Read the model definition and answer for the solid it produces. Units are mm, in the model's axes. Face numbers are marked on the shaded views. Coordinates: 2 decimals unless noted, no trailing zeros. Loops run counter-clockwise (first coordinate to the right, second up) from the corner with the lowest first, then second, coordinate; pieces in that order, holes last. Notation, with made-up numbers: (38.5, -8.5) -> (84.5, -8.5) arc R23 ccw to (84.5, 4.5) -> close; hole circle Ø11 at (14.5, -25). An arc over 180 degrees is marked (long way). Answer as a JSON object with one key per item and string values. Group by question number.
1) Flat-ended cylindrical pins translate along their axes: P1, Ø1.5, axis at y = 5.5, z = 7.5, coming from the -X side; P2, Ø2, axis at x = 5, y = 1, coming from the +Z side. Find the tip coordinate at first contact, or state that the pin passes through.
2) Determine the mould class of the marked faces 1, 2 and 3 for opening direction X: released by +X, released by -X, zero draft, split by the parting line, or undercut.
3) Section D-D, the plane z = 7.5 is taken. Give the vertices of the cut face in (x, y), plus the area to 3 significant figures.
4) Section C-C, the plane y = 1.75 is taken. Give the vertices of the cut face in (x, z), plus the area to 3 significant figures.
5) Section B-B, the plane z = 0 is taken. Give the vertices of the cut face in (x, y).
6) Consider probe 1 along Z at (x, y) = (0, 3.25); probe 2 along X at (y, z) = (5.25, 0.5); probe 3 along Z at (x, y) = (1.25, 2). Determine where each line is inside the solid, lowest interval first. Write a range as [from, to].
7) Section A-A, the plane x = 8 is taken. Give the vertices of the cut face in (y, z).
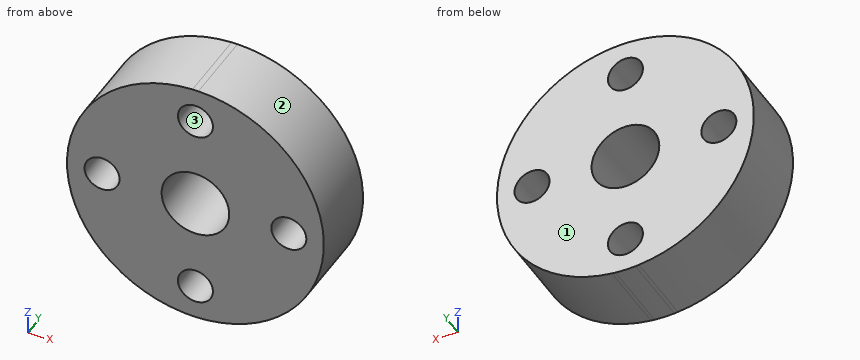
Autodesk Inventor part; units mm, degrees
ref_plane "YZ Plane" through (0, 0, 0) normal (1, 0, 0) x (0, 1, 0)
ref_plane "XZ Plane" through (0, 0, 0) normal (0, 1, 0) x (-1, 0, 0)
ref_plane "XY Plane" through (0, 0, 0) normal (0, 0, 1) x (1, 0, 0)
sketch "Эскиз1" plane through (0, 0, 0) normal (0, 1, 0) x (-1, 0, 0)
  arc A0 (-0.25, 9.2247) -> (0.25, 9.2247) centre (0, 8) ccw
  line L0 (-0.25, 10.9972) -> (-0.25, 9.2247)
  arc A1 (-0.25, 10.9972) -> (-1.1469, -10.94) centre (0, 0) ccw
  line L1 (-1.1469, -10.6297) -> (-1.1469, -10.94)
  line L2 (-0.8473, -10.6297) -> (-1.1469, -10.6297)
  line L3 (-0.8473, -10.9673) -> (-0.8473, -10.6297)
  arc A2 (-0.8473, -10.9673) -> (0.8535, -10.9668) centre (0, 0) ccw
  line L4 (0.8535, -10.6297) -> (0.8535, -10.9668)
  line L5 (1.1541, -10.6297) -> (0.8535, -10.6297)
  line L6 (1.1541, -10.9393) -> (1.1541, -10.6297)
  arc A3 (1.1541, -10.9393) -> (0.25, 10.9972) centre (0, 0) ccw
  line L7 (0.25, 9.2247) -> (0.25, 10.9972)
  circle A4 centre (8, 0) radius 1.25
  circle A5 centre (0, -8) radius 1.25
  circle A6 centre (-8, 0) radius 1.25
  circle A7 centre (0, -5.5) radius 0.75
  circle A8 centre (4.7631, 2.75) radius 0.75
  circle A9 centre (-4.7631, 2.75) radius 0.75
  circle A10 centre (0, 0) radius 2.9
  arc A11 (0.25, 9.2247) -> (-0.25, 9.2247) centre (0, 8) ccw
  line L8 (0.25, 10.9972) -> (-0.25, 10.9972)
  line L9 (1.1541, -10.9393) -> (0.8535, -10.9668)
  line L10 (-0.8473, -10.9673) -> (-1.1541, -10.9393)
extrude "Выдавливание1" add sketch "Эскиз1" along normal blind 6.5 contours A0 L7 A3 L6 L5 L4 A2 L3 L2 L1 A1 L0 | L0 L8 L7 A11 | L9 L4 L5 L6 | L1 L2 L3 L10 | A7 | A8 | A9
sketch "Эскиз2" plane through (0, 6.5, 0) normal (0, 1, 0) x (1, 0, 0)
  circle A0 centre (0, -8) radius 1.25
  circle A1 centre (0, -8) radius 1.5
  circle A2 centre (-8, 0) radius 1.25
  circle A3 centre (-8, 0) radius 1.5
  circle A4 centre (0, 8) radius 1.25
  circle A5 centre (0, 8) radius 1.5
  circle A6 centre (8, 0) radius 1.25
  circle A7 centre (8, 0) radius 1.5
  point P0 (0, 0)
  dimension "d2" = 3
  dimension "d3" = 3
  dimension "d4" = 3
  dimension "d5" = 3
extrude "Выдавливание2" cut sketch "Эскиз2" against normal blind 10 contours A0 | A1 | A2 | A3 | A4 | A5 | A6 | A7
properties part number "проставка"
Determined:
{
 "1": {"P1": "x = -8.69", "P2": "z = 10.25"},
 "2": {"face 1": "zero draft", "face 2": "released by +X", "face 3": "undercut"},
 "3": {"outline": "(-8.05, 0) -> (-1.41, 0) -> (-1.41, 6.5) -> (-8.05, 6.5) -> close; (1.41, 0) -> (8.05, 0) -> (8.05, 6.5) -> (1.41, 6.5) -> close", "area": "86.2 mm²"},
 "4": {"outline": "(-1.15, -10.94) -> (-0.85, -10.97) arc R11 ccw to (0.85, -10.97) -> (1.15, -10.94) arc R11 ccw to (0.25, 11) -> (-0.25, 11) arc R11 ccw to start; hole circle Ø3 at (-8, 0); hole circle Ø5.8 at (0, 0); hole circle Ø3 at (0, -8); hole circle Ø3 at (0, 8); hole circle Ø3 at (8, 0)", "area": "325 mm²"},
 "5": {"outline": "(-11, 0) -> (-9.5, 0) -> (-9.5, 6.5) -> (-11, 6.5) -> close; (-6.5, 0) -> (-2.9, 0) -> (-2.9, 6.5) -> (-6.5, 6.5) -> close; (2.9, 0) -> (6.5, 0) -> (6.5, 6.5) -> (2.9, 6.5) -> close; (9.5, 0) -> (11, 0) -> (11, 6.5) -> (9.5, 6.5) -> close"},
 "6": {"probe 1": "[-11, -9.5], [-6.5, -2.9], [2.9, 6.5], [9.5, 11]", "probe 2": "[-10.99, -9.41], [-6.59, -2.86], [2.86, 6.59], [9.41, 10.99]", "probe 3": "[-10.93, -8.83], [-7.17, -2.62], [2.62, 7.17], [8.83, 10.93]"},
 "7": {"outline": "(0, -7.55) -> (6.5, -7.55) -> (6.5, -1.5) -> (0, -1.5) -> close; (0, 1.5) -> (6.5, 1.5) -> (6.5, 7.55) -> (0, 7.55) -> close"}
}
